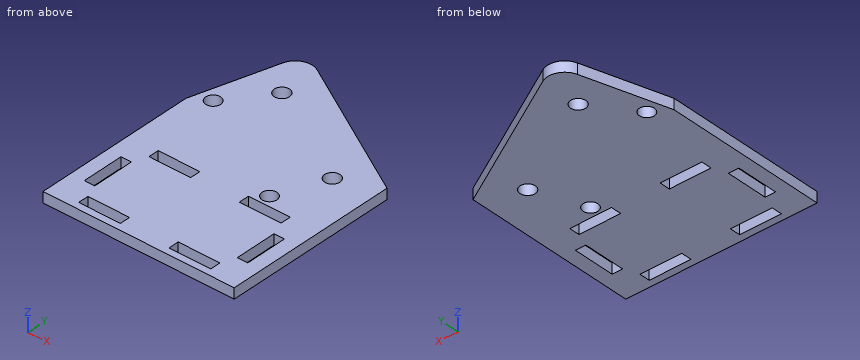
```python
from build123d import *

# Parameters (mm, degrees)
SKETCH_1_W          = 55
SKETCH_1_H          = 30
EXTRUDE_1_DEPTH     = 3
SKETCH_2_W          = 12
SKETCH_2_H          = 3
SKETCH_2_W_2        = 3
SKETCH_2_H_2        = 12
CUT_EXTRUDE_1_DEPTH = 3
SKETCH_3_R          = 2.2
CUT_EXTRUDE_2_DEPTH = 10
CUT_EXTRUDE_3_DEPTH = 10
FILLET_1_R          = 5
SKETCH_5_R          = 2.15
CUT_EXTRUDE_4_DEPTH = 3


with BuildPart() as part:
    # 草图1 → 凸台-拉伸1 (new body)
    with BuildSketch(Plane.XY):
        Polygon((27.5, 35), (-27.5, 66.754264805), (-27.5, 15), (27.5, 15), align=None)
        Rectangle(SKETCH_1_W, SKETCH_1_H)
    extrude(amount=EXTRUDE_1_DEPTH)

    # 草图2 → 切除-拉伸1 (cut)
    with BuildSketch(Plane.XY.offset(3)):
        with Locations((-13, -11.5)):
            Rectangle(SKETCH_2_W, SKETCH_2_H)
        with Locations((13, -11.5)):
            Rectangle(SKETCH_2_W, SKETCH_2_H)
        with Locations((13, 11.5)):
            Rectangle(SKETCH_2_W, SKETCH_2_H)
        with Locations((-13, 11.5)):
            Rectangle(SKETCH_2_W, SKETCH_2_H)
        with Locations((22, 0)):
            Rectangle(SKETCH_2_W_2, SKETCH_2_H_2)
        with Locations((-22, 0)):
            Rectangle(SKETCH_2_W_2, SKETCH_2_H_2)
    extrude(amount=-CUT_EXTRUDE_1_DEPTH, mode=Mode.SUBTRACT)

    # 草图3 → 切除-拉伸2 (cut)
    with BuildSketch(Plane.XY.offset(3)):
        with Locations((-13.284609691, 47)):
            Circle(SKETCH_3_R)
        with Locations((16.160254038, 30)):
            Circle(SKETCH_3_R)
    extrude(amount=-CUT_EXTRUDE_2_DEPTH, mode=Mode.SUBTRACT)

    # 草图4 → 切除-拉伸3 (cut)
    with BuildSketch(Plane.XY.offset(3)):
        Polygon((-18.839745962, 61.754264805), (-27.5, 31.754264805), (-27.5, 66.754264805), align=None)
    extrude(amount=-CUT_EXTRUDE_3_DEPTH, mode=Mode.SUBTRACT)

    # 圆角1
    fillet_1_edges = [part.edges().sort_by_distance(p)[0] for p in [
        (-18.839745962, 61.754264805, 1.5),
    ]]
    fillet(fillet_1_edges, radius=FILLET_1_R)

    # 草图5 → 切除-拉伸4 (cut)
    with BuildSketch(Plane(origin=(0, 0, 0), x_dir=(-1, 0, 0), z_dir=(0, 0, -1))):
        with Locations((-10.392304845, 16.009618943)):
            Circle(SKETCH_5_R)
        with Locations((22.516660498, 35.009618943)):
            Circle(SKETCH_5_R)
    extrude(amount=-CUT_EXTRUDE_4_DEPTH, mode=Mode.SUBTRACT)


solid = part.part
```
Geometry: final body of the model. Coordinates: model frame, mm. Round coordinates to 2 decimals unless told otherwise and drop trailing zeros. Order: outer loops, then holes, each group sorted by start corner. A loop starts at its lowest first (then second) coordinate and runs counter-clockwise, first axis right, second up. Notation, with made-up numbers: (1, 56.5) -> (32, 56.5) arc R9 ccw to (32, 68.5) -> close; hole circle Ø8 at (18.5, -40). An arc over 180 degrees is marked (long way). Write each question's results on one line, items separated by ' | '.
Q1. Section query A-A (y = 1.5). Output: boundary loops of the cut face in (x, z), and give its area (3 significant figures).
Response values:
outline: (-27.5, 0) -> (-23.5, 0) -> (-23.5, 3) -> (-27.5, 3) -> close; (-20.5, 0) -> (20.5, 0) -> (20.5, 3) -> (-20.5, 3) -> close; (23.5, 0) -> (27.5, 0) -> (27.5, 3) -> (23.5, 3) -> close | area: 147 mm²
Q2. Section query C-C (z = 1.3). Count the separate pieces of the cut face and the enclosed holes in it, and give its area (3 significant figures).
Response values:
separate pieces: 1 | enclosed holes: 10 | area: 3,190 mm²
Q3. Ray query, line 1 along X through (y, z) = (-1, 2.2); line 2 along Y through (x, z) = (-8, 0.5); line 3 along Y through (x, z) = (11.5, 2.05). Return the intervals inside material, ascending.
Response values:
line 1: -27.5 to -23.5, -20.5 to 20.5, 23.5 to 27.5 | line 2: -15 to -13, -10 to 10, 13 to 55.5 | line 3: -15 to -13, -10 to 10, 13 to 14.17, 17.85 to 44.24
Q4. Pin query (flat end, axial travel): pin 1 Ø1.5 at (x, z) = (13, 2) entering from +Y. Return the tip coordinate at first contact, or that it passes through.
Response values:
pin 1: y = 43.8
Q5. Section query B-B (y = 30). Output: boundary loops of the cut face in (x, z).
Response values:
outline: (-27.5, 0) -> (13.96, 0) -> (13.96, 3) -> (-27.5, 3) -> close; (18.36, 0) -> (27.5, 0) -> (27.5, 3) -> (18.36, 3) -> close
Q6. Section query D-D (y = 47). Output: boundary loops of the cut face in (x, z), and give its area (3 significant figures).
Response values:
outline: (-23.1, 0) -> (-15.48, 0) -> (-15.48, 3) -> (-23.1, 3) -> close; (-11.08, 0) -> (6.72, 0) -> (6.72, 3) -> (-11.08, 3) -> close | area: 76.2 mm²
